from build123d import *

# Parameters (mm, degrees)
F0_R     = 3.175
F1_DEPTH = 6.35


with BuildPart() as f1:
    # F0 (on Front) → F1 (new body)
    with BuildSketch(Plane.XZ):
        with BuildLine():
            ThreePointArc((19.019852, -1.071327), (19.042461, -0.535875), (19.05, 0))
            ThreePointArc((19.05, 0), (19.037896, 0.678973), (19.001601, 1.357083))
            ThreePointArc((19.001601, 1.357083), (18.539994, 4.378484), (17.601125, 7.287173))
            ThreePointArc((17.601125, 7.287173), (17.100853, 8.394243), (16.531034, 9.467175))
            ThreePointArc((16.531034, 9.467175), (14.804204, 11.98908), (12.69628, 14.202358))
            ThreePointArc((12.69628, 14.202358), (11.765211, 14.982734), (10.786294, 15.702177))
            ThreePointArc((10.786294, 15.702177), (8.136261, 17.225091), (5.276781, 18.304592))
            ThreePointArc((5.276781, 18.304592), (4.099324, 18.60371), (2.905195, 18.82717))
            ThreePointArc((2.905195, 18.82717), (-0.14317, 19.049462), (-3.187849, 18.781377))
            ThreePointArc((-3.187849, 18.781377), (-4.378484, 18.539994), (-5.551312, 18.223211))
            ThreePointArc((-5.551312, 18.223211), (-8.394243, 17.100853), (-11.021087, 15.53828))
            ThreePointArc((-11.021087, 15.53828), (-11.98908, 14.804204), (-12.908315, 14.009922))
            ThreePointArc((-12.908315, 14.009922), (-14.982734, 11.765211), (-16.671463, 9.217636))
            ThreePointArc((-16.671463, 9.217636), (-17.225091, 8.136261), (-17.708667, 7.021796))
            ThreePointArc((-17.708667, 7.021796), (-18.60371, 4.099324), (-19.019852, 1.071327))
            ThreePointArc((-19.019852, 1.071327), (-19.049462, -0.14317), (-19.001601, -1.357083))
            ThreePointArc((-19.001601, -1.357083), (-18.539994, -4.378484), (-17.601125, -7.287173))
            ThreePointArc((-17.601125, -7.287173), (-17.100853, -8.394243), (-16.531034, -9.467175))
            ThreePointArc((-16.531034, -9.467175), (-14.804204, -11.98908), (-12.69628, -14.202358))
            ThreePointArc((-12.69628, -14.202358), (-11.765211, -14.982734), (-10.786294, -15.702177))
            ThreePointArc((-10.786294, -15.702177), (-8.136261, -17.225091), (-5.276781, -18.304592))
            ThreePointArc((-5.276781, -18.304592), (-4.099324, -18.60371), (-2.905195, -18.82717))
            ThreePointArc((-2.905195, -18.82717), (0.14317, -19.049462), (3.187849, -18.781377))
            ThreePointArc((3.187849, -18.781377), (4.378484, -18.539994), (5.551312, -18.223211))
            ThreePointArc((5.551312, -18.223211), (8.394243, -17.100853), (11.021087, -15.53828))
            ThreePointArc((11.021087, -15.53828), (11.98908, -14.804204), (12.908315, -14.009922))
            ThreePointArc((12.908315, -14.009922), (14.982734, -11.765211), (16.671463, -9.217636))
            ThreePointArc((16.671463, -9.217636), (17.225091, -8.136261), (17.708667, -7.021796))
            ThreePointArc((17.708667, -7.021796), (18.60371, -4.099324), (19.019852, -1.071327))
        make_face()
        Circle(F0_R, mode=Mode.SUBTRACT)
        with BuildLine():
            ThreePointArc((17.601125, 7.287173), (18.539994, 4.378484), (19.001601, 1.357083))
            Line((19.001601, 1.357083), (21.347045, 3.497063))
            Line((21.347045, 3.497063), (20.668801, 6.468644))
            Line((20.668801, 6.468644), (17.601125, 7.287173))
        make_face()
        with BuildLine():
            Line((21.428586, -3.13981), (19.019852, -1.071327))
            ThreePointArc((19.019852, -1.071327), (18.60371, -4.099324), (17.708667, -7.021796))
            Line((17.708667, -7.021796), (20.750342, -6.11139))
            Line((20.750342, -6.11139), (21.428586, -3.13981))
        make_face()
        with BuildLine():
            ThreePointArc((12.69628, 14.202358), (14.804204, 11.98908), (16.531034, 9.467175))
            Line((16.531034, 9.467175), (17.715704, 12.412881))
            Line((17.715704, 12.412881), (15.815307, 14.795903))
            Line((15.815307, 14.795903), (12.69628, 14.202358))
        make_face()
        with BuildLine():
            Line((17.944176, -12.126386), (16.671463, -9.217636))
            ThreePointArc((16.671463, -9.217636), (14.982734, -11.765211), (12.908315, -14.009922))
            Line((12.908315, -14.009922), (16.043779, -14.509409))
            Line((16.043779, -14.509409), (17.944176, -12.126386))
        make_face()
        with BuildLine():
            ThreePointArc((5.276781, 18.304592), (8.136261, 17.225091), (10.786294, 15.702177))
            Line((10.786294, 15.702177), (10.575551, 18.870175))
            Line((10.575551, 18.870175), (7.829398, 20.192653))
            Line((7.829398, 20.192653), (5.276781, 18.304592))
        make_face()
        with BuildLine():
            Line((10.905702, -18.711183), (11.021087, -15.53828))
            ThreePointArc((11.021087, -15.53828), (8.394243, -17.100853), (5.551312, -18.223211))
            Line((5.551312, -18.223211), (8.159549, -20.03366))
            Line((8.159549, -20.03366), (10.905702, -18.711183))
        make_face()
        with BuildLine():
            ThreePointArc((-3.187849, 18.781377), (-0.14317, 19.049462), (2.905195, 18.82717))
            Line((2.905195, 18.82717), (1.34078, 21.59))
            Line((1.34078, 21.59), (-1.70722, 21.59))
            Line((-1.70722, 21.59), (-3.187849, 18.781377))
        make_face()
        with BuildLine():
            Line((1.70722, -21.59), (3.187849, -18.781377))
            ThreePointArc((3.187849, -18.781377), (0.14317, -19.049462), (-2.905195, -18.82717))
            Line((-2.905195, -18.82717), (-1.34078, -21.59))
            Line((-1.34078, -21.59), (1.70722, -21.59))
        make_face()
        with BuildLine():
            ThreePointArc((-11.021087, 15.53828), (-8.394243, 17.100853), (-5.551312, 18.223211))
            Line((-5.551312, 18.223211), (-8.159549, 20.03366))
            Line((-8.159549, 20.03366), (-10.905702, 18.711183))
            Line((-10.905702, 18.711183), (-11.021087, 15.53828))
        make_face()
        with BuildLine():
            Line((-7.829398, -20.192653), (-5.276781, -18.304592))
            ThreePointArc((-5.276781, -18.304592), (-8.136261, -17.225091), (-10.786294, -15.702177))
            Line((-10.786294, -15.702177), (-10.575551, -18.870175))
            Line((-10.575551, -18.870175), (-7.829398, -20.192653))
        make_face()
        with BuildLine():
            ThreePointArc((-16.671463, 9.217636), (-14.982734, 11.765211), (-12.908315, 14.009922))
            Line((-12.908315, 14.009922), (-16.043779, 14.509409))
            Line((-16.043779, 14.509409), (-17.944176, 12.126386))
            Line((-17.944176, 12.126386), (-16.671463, 9.217636))
        make_face()
        with BuildLine():
            Line((-15.815307, -14.795903), (-12.69628, -14.202358))
            ThreePointArc((-12.69628, -14.202358), (-14.804204, -11.98908), (-16.531034, -9.467175))
            Line((-16.531034, -9.467175), (-17.715704, -12.412881))
            Line((-17.715704, -12.412881), (-15.815307, -14.795903))
        make_face()
        with BuildLine():
            ThreePointArc((-19.019852, 1.071327), (-18.60371, 4.099324), (-17.708667, 7.021796))
            Line((-17.708667, 7.021796), (-20.750342, 6.11139))
            Line((-20.750342, 6.11139), (-21.428586, 3.13981))
            Line((-21.428586, 3.13981), (-19.019852, 1.071327))
        make_face()
        with BuildLine():
            Line((-20.668801, -6.468644), (-17.601125, -7.287173))
            ThreePointArc((-17.601125, -7.287173), (-18.539994, -4.378484), (-19.001601, -1.357083))
            Line((-19.001601, -1.357083), (-21.347045, -3.497063))
            Line((-21.347045, -3.497063), (-20.668801, -6.468644))
        make_face()
    extrude(amount=F1_DEPTH)


solid = f1.part
Design review of the part built by this model. Coordinates are the model's own, in mm. A direction names the side the tool comes from. Round coordinates to 2 decimals unless told otherwise and drop trailing zeros. Write each loop counter-clockwise with the first axis right and the second up, starting at its lowest first coordinate (ties: lowest second). Pieces come first, ordered by that corner, then holes.
Item 1: Consider section C-C on x = 9. Give the boundary of the cut face in (y, z), and give its area (3 significant figures).
Item 2: Consider section B-B on z = 11.5. Give the boundary of the cut face in (x, y), and give its area (3 significant figures).
Item 3: For pin 1 Ø5 at (x, z) = (0, 0) entering from +Y; pin 2 Ø3 at (x, y) = (-3.5, -3.5) entering from -Z; pin 3 Ø3 at (y, z) = (-1.5, -15.5) entering from +X; pin 4 Ø2 at (y, z) = (-5, -16.5) entering from -X, all flat-tipped, find the tip position at first contact; note any pin that passes through.
Item 4: Consider section A-A on x = 0. Give the boundary of the cut face in (y, z) (3 decimals).
Item 5: Wall thickness on L1, parallel to Z at x = 0, y = -2.25 (3 decimals); L2, parallel to Z at x = -0.5, y = -4.5; L3, parallel to X at y = -0.25, z = 3.5: over which ranges is each line inside the solid? List them lowest first.
Item 6: For faces 1 (the cylindrical face through (-17.1, -3.1, -8.4)), 2 (the flat face through (14.278, -3.131, 14.503)), 3 (the flat face through (17.115, -3.131, 10.919)), 4 (the flat face through (-6.57, -3.13, -19.26)), list the 3-axis set-ups (+Z, -Z, +X, -X, +Y, -Y) from which the entire face can be reached by the end or side of a thin tool; tool diameter is ignored.
Check values:
1. outline: (-6.35, -19.63) - (0, -19.63) - (0, 19.63) - (-6.35, 19.63) - close
1. area: 249 mm2
2. outline: (-17.67, -6.35) - (17.35, -6.35) - (17.35, 0) - (-17.67, 0) - close
2. area: 222 mm2
3. pin 1: passes through
3. pin 2: stops at z = -20.43
3. pin 3: stops at x = 16.45
3. pin 4: stops at x = -11.07
4. outline: (-6.35, -21.59) - (0, -21.59) - (0, -3.175) - (-6.35, -3.175) - close; (-6.35, 3.175) - (0, 3.175) - (0, 21.59) - (-6.35, 21.59) - close
5. L1: z = -21.59 to -3.175, 3.175 to 21.59
5. L2: z = -21.59 to -3.14, 3.14 to 21.59
5. L3: x = -21.35 to 21.35
6. face 1: -X, +Y, -Y
6. face 2: +Z, +Y, -Y
6. face 3: +X, +Y, -Y
6. face 4: -Z, +Y, -Y
